Build history of the part. All positions in model axes, mm. A direction names the side the tool comes from. Give positions to 0.01 mm unless a question says otherwise; leave off trailing zeros. Loops run counter-clockwise (first coordinate to the right, second up) from the corner with the lowest first, then second, coordinate; pieces in that order, holes last.
1) Wall check: line 1 (Y direction, x = 0, z = 20); line 2 (Z direction, x = -6.25, y = -4). Give the ranges that are in metal, low to high.
2) Flat gauge pins, fed straight in: P1, Ø3, axis at x = 2, y = 8, coming from the -Z side; P2, Ø0.8, axis at x = 7, z = 0.5, coming from the -Y side; P3, Ø1.6, axis at x = 7, z = 1, coming from the +Y side. Where does each tip first touch, or does it go through?
3) Band-saw the part on B-B on z = 12. List the corners of the cut face in (x, y).
4) Band-saw the part on A-A on x = 6.75. List the corners of the cut face in (y, z), then the cut area to 3 significant figures.
5) 3-axis set-ups, long thin cutter, end or side, ignore diameter. For faces 1 (the flat face through (7, -1.25, 1)), 2 (the flat face through (-6, 6, 30)), 3 (the flat face through (-7, 1.25, 1)): which of +Z, -Z, +X, -X, +Y, -Y reach the whole face in a straight line?
6) Two-plate mould, pull along X, no slides. Class faces 4 (the cylindrical face through (-0.13, -11.01, 32.47)), 5 (the cylindrical face through (9.599, 5.396, 32.465)), 6 (the cylindrical face through (-6.46, -10.7, 32.47)): +X half, -X half, draft (parallel to the pull), parting line (faces both ways), or undercut.
```python
from build123d import *

# Parameters (mm, degrees)
SKETCH1_R               = 8
SKETCH1_R_2             = 6.05
BOSS_EXTRUDE1_DEPTH     = 30
CUT_EXTRUDE1_DEPTH      = 33.062439084
CUT_EXTRUDE1_DEPTH_BACK = 33.062439084
SKETCH2_W               = 6.75
SKETCH2_H               = 1.5
SKETCH3_R               = 12.5
SKETCH3_R_2             = 6.05
BOSS_EXTRUDE2_DEPTH     = 5
CUT_EXTRUDE2_DEPTH      = 40.210967853
CUT_EXTRUDE2_DEPTH_BACK = 40.210967853
SKETCH4_R               = 4


with BuildPart() as part:
    # Sketch1 → Boss-Extrude1 (new body)
    with BuildSketch(Plane(origin=(0, 0, 0), x_dir=(0, 1, 0), z_dir=(0, 0, 1))):
        with Locations(Location((0, 0, 0), (0, 0, 270))):
            Circle(SKETCH1_R)
        with Locations(Location((0, 0, 0), (0, 0, 270))):
            Circle(SKETCH1_R_2, mode=Mode.SUBTRACT)
    extrude(amount=BOSS_EXTRUDE1_DEPTH)

    # Sketch2 → Cut-Extrude1 (cut, two sides: drawn at the far end of the back side and taken through both)
    with BuildSketch(Plane.YZ.offset(-CUT_EXTRUDE1_DEPTH_BACK)):
        with Locations((-4.625, 0.75)):
            Rectangle(SKETCH2_W, SKETCH2_H)
        with Locations((4.625, 0.75)):
            Rectangle(SKETCH2_W, SKETCH2_H)
    extrude(amount=CUT_EXTRUDE1_DEPTH + CUT_EXTRUDE1_DEPTH_BACK, mode=Mode.SUBTRACT)

    # Sketch3 → Boss-Extrude2 (add)
    with BuildSketch(Plane.XY.offset(30)):
        Circle(SKETCH3_R)
        with Locations(Location((0, 0, 0), (0, 0, 168.076144872))):
            Circle(SKETCH3_R_2, mode=Mode.SUBTRACT)
    extrude(amount=BOSS_EXTRUDE2_DEPTH)

    # Sketch4 → Cut-Extrude2 (cut, two sides: drawn at the far end of the back side and taken through both)
    with BuildSketch(Plane.XY.offset(35).offset(-CUT_EXTRUDE2_DEPTH_BACK)):
        with Locations((-12.882183606, 7.706015759)):
            Circle(SKETCH4_R)
        with Locations((0.232513607, 15.009306138)):
            Circle(SKETCH4_R)
        with Locations((13.114697212, 7.303290379)):
            Circle(SKETCH4_R)
        with Locations((12.882183606, -7.706015759)):
            Circle(SKETCH4_R)
        with Locations((-0.232513607, -15.009306138)):
            Circle(SKETCH4_R)
        with Locations((-13.114697212, -7.303290379)):
            Circle(SKETCH4_R)
    extrude(amount=CUT_EXTRUDE2_DEPTH + CUT_EXTRUDE2_DEPTH_BACK, mode=Mode.SUBTRACT)


solid = part.part
```
Findings below:
1. line 1: y = -8 to -6.05, 6.05 to 8
1. line 2: z = 1.5 to 35
2. P1: stops at z = 1.5
2. P2: stops at y = -1.25
2. P3: stops at y = 4.83
3. outline: circle Ø16 at (0, 0); hole circle Ø12.1 at (0, 0)
4. outline: (-10.52, 30) - (-4.29, 30) - (-4.29, 1.5) - (-1.25, 1.5) - (-1.25, 0) - (1.25, 0) - (1.25, 1.5) - (4.29, 1.5) - (4.29, 30) - (10.52, 30) - (10.52, 35) - (-10.52, 35) - close
4. area: 354 mm2
5. face 1: -Z, +X, -X, -Y
5. face 2: -Z
5. face 3: -Z, +X, -X, +Y
6. face 4: undercut
6. face 5: +X half
6. face 6: -X half
